Can you work these out from the model? Positions are in its coordinate system, mm. A direction names the side the tool comes from. Coordinates: 2 decimals unless noted, no trailing zeros. Loops run counter-clockwise (first coordinate to the right, second up) from the corner with the lowest first, then second, coordinate; pieces in that order, holes last. Notation, with made-up numbers: (-6.5, 38) -> (51.5, 38) arc R20 ccw to (51.5, 67) -> close; hole circle Ø7 at (-11.75, 21). An arc over 180 degrees is marked (long way). Use one line per item in the form item = value. Start each with the question number.
(1) On a 3-axis mill with a long thin cutter (end or side, diameter ignored), from which of +Z, -Z, +X, -X, +Y, -Y can I reach the whole of each face in a straight line? I mean faces 1 (the flat face through (3, -17.5, -124)), 2 (the cylindrical face through (-2.75, -92.74, 20.59)), 3 (the flat face through (3, 17.5, 124)). Say none if no direction works.
(2) Imagine slicing it at D-D (z = -121.5). List the corners of the cut face in (x, y) for me, plus the area to 3 significant figures.
(3) Thinking about a two-plate mould opening in Y: for faces 4 (the flat face through (3.41, 115.96, -46.74)), 5 (the flat face through (10, 59.85, 45.49)), 6 (the flat face through (0, 76, 0)), 7 (the cylindrical face through (3.409, 121.16, -60.934)), which applies, released by +Y, released by -Y, zero draft, split by the parting line, or undercut?
(4) I need wall thicknesses on line 1 (Y direction, x = 7.5, z = -62); line 2 (Y direction, x = 5, z = 75.5); line 3 (Y direction, x = -2.8, z = 0). Which ranges of each line are inside material? Lowest first, please. Write a range as [from, to].
(5) I'm going to push flat-ended pins straight in: pin 1 (4 mm diameter, centred on x = 6, z = -45.5, fed in from +Y); pin 2 (18.5 mm diameter, centred on y = 0, z = 133.66, fed in from -X); pin 3 (14.5 mm diameter, centred on y = 115.75, z = 66.83, fed in from -X); pin 4 (2 mm diameter, centred on y = -61.5, z = 56, fed in from -X). Where does each tip first touch, or does it pass through?
(6) Imagine slicing it at A-A (y = 0). List the corners of the cut face in (x, z) for me, plus the area to 3 significant figures.
(7) Imagine slicing it at C-C (x = 4.25). State how many separate pieces and enclosed holes the cut face has, plus the area to 3 significant figures.
(8) Imagine slicing it at B-B (z = 0). List the corners of the cut face in (x, y) for me, plus the area to 3 significant figures.
```python
from build123d import *

# Parameters (mm, degrees)
SKETCH2_R           = 115
SKETCH2_R_2         = 95
SKETCH2_R_3         = 75
SKETCH2_R_4         = 8
BOSS_EXTRUDE1_DEPTH = 10
BOSS_EXTRUDE2_START = -3
SKETCH2_5_R         = 115
SKETCH2_5_R_2       = 95
SKETCH2_5_R_3       = 8
BOSS_EXTRUDE2_DEPTH = 3
FILLET1_R           = 2.5


with BuildPart() as part:
    # Sketch2 → Boss-Extrude1 (new body)
    # profile 1 of 8: a face of its own
    with BuildSketch(Plane(origin=(0, 0, 0), x_dir=(0, 0, -1), z_dir=(1, 0, 0))):
        Circle(SKETCH2_R)
        Circle(SKETCH2_R_2, mode=Mode.SUBTRACT)
    # profile 2 of 8: a face of its own
    with BuildSketch(Plane(origin=(0, 0, 0), x_dir=(0, 0, -1), z_dir=(1, 0, 0))):
        Circle(SKETCH2_R_2)
        Circle(SKETCH2_R_3, mode=Mode.SUBTRACT)
    # profile 3 of 8: a face of its own
    with BuildSketch(Plane(origin=(0, 0, 0), x_dir=(0, 0, -1), z_dir=(1, 0, 0))):
        with BuildLine():
            ThreePointArc((-113.660679217, -17.5), (-115, 0), (-113.660679217, 17.5))
            Line((-113.660679217, 17.5), (-133.660679217, 17.5))
            ThreePointArc((-133.660679217, 17.5), (-151.160679217, 0), (-133.660679217, -17.5))
            Line((-133.660679217, -17.5), (-113.660679217, -17.5))
        make_face()
        with Locations((-133.660679217, 0)):
            Circle(SKETCH2_R_4, mode=Mode.SUBTRACT)
    # profile 4 of 8: a face of its own
    with BuildSketch(Plane(origin=(0, 0, 0), x_dir=(0, 0, -1), z_dir=(1, 0, 0))):
        with BuildLine():
            ThreePointArc((-71.985784175, 89.683035613), (-57.5, 99.592921435), (-41.674895042, 107.183035613))
            Line((-41.674895042, 107.183035613), (-51.674895042, 124.503543689))
            ThreePointArc((-51.674895042, 124.503543689), (-75.580339608, 130.908988255), (-81.985784175, 107.003543689))
            Line((-81.985784175, 107.003543689), (-71.985784175, 89.683035613))
        make_face()
        with Locations((-66.830339608, 115.753543689)):
            Circle(SKETCH2_R_4, mode=Mode.SUBTRACT)
    # profile 5 of 8: a face of its own
    with BuildSketch(Plane(origin=(0, 0, 0), x_dir=(0, 0, -1), z_dir=(1, 0, 0))):
        with BuildLine():
            ThreePointArc((41.674895042, 107.183035613), (57.5, 99.592921435), (71.985784175, 89.683035613))
            Line((71.985784175, 89.683035613), (81.985784175, 107.003543689))
            ThreePointArc((81.985784175, 107.003543689), (75.580339608, 130.908988255), (51.674895042, 124.503543689))
            Line((51.674895042, 124.503543689), (41.674895042, 107.183035613))
        make_face()
        with Locations((66.830339608, 115.753543689)):
            Circle(SKETCH2_R_4, mode=Mode.SUBTRACT)
    # profile 6 of 8: a face of its own
    with BuildSketch(Plane(origin=(0, 0, 0), x_dir=(0, 0, -1), z_dir=(1, 0, 0))):
        with BuildLine():
            Line((133.660679217, 17.5), (113.660679217, 17.5))
            ThreePointArc((113.660679217, 17.5), (114.66468094, 8.775588017), (115, 0))
            ThreePointArc((115, 0), (114.66468094, -8.775588017), (113.660679217, -17.5))
            Line((113.660679217, -17.5), (133.660679217, -17.5))
            ThreePointArc((133.660679217, -17.5), (151.160679217, 0), (133.660679217, 17.5))
        make_face()
        with Locations((133.660679217, 0)):
            Circle(SKETCH2_R_4, mode=Mode.SUBTRACT)
    # profile 7 of 8: a face of its own
    with BuildSketch(Plane(origin=(0, 0, 0), x_dir=(0, 0, -1), z_dir=(1, 0, 0))):
        with BuildLine():
            Line((81.985784175, -107.003543689), (71.985784175, -89.683035613))
            ThreePointArc((71.985784175, -89.683035613), (57.5, -99.592921435), (41.674895042, -107.183035613))
            Line((41.674895042, -107.183035613), (51.674895042, -124.503543689))
            ThreePointArc((51.674895042, -124.503543689), (75.580339608, -130.908988255), (81.985784175, -107.003543689))
        make_face()
        with Locations((66.830339608, -115.753543689)):
            Circle(SKETCH2_R_4, mode=Mode.SUBTRACT)
    # profile 8 of 8: a face of its own
    with BuildSketch(Plane(origin=(0, 0, 0), x_dir=(0, 0, -1), z_dir=(1, 0, 0))):
        with BuildLine():
            Line((-51.674895042, -124.503543689), (-41.674895042, -107.183035613))
            ThreePointArc((-41.674895042, -107.183035613), (-57.5, -99.592921435), (-71.985784175, -89.683035613))
            Line((-71.985784175, -89.683035613), (-81.985784175, -107.003543689))
            ThreePointArc((-81.985784175, -107.003543689), (-75.580339608, -130.908988255), (-51.674895042, -124.503543689))
        make_face()
        with Locations((-66.830339608, -115.753543689)):
            Circle(SKETCH2_R_4, mode=Mode.SUBTRACT)
    extrude(amount=BOSS_EXTRUDE1_DEPTH)

    # Sketch2_5 → Boss-Extrude2 (add)
    # profile 1 of 7: a face of its own
    with BuildSketch(Plane(origin=(0, 0, 0), x_dir=(0, 0, -1), z_dir=(1, 0, 0)).offset(BOSS_EXTRUDE2_START)):
        Circle(SKETCH2_5_R)
        Circle(SKETCH2_5_R_2, mode=Mode.SUBTRACT)
    # profile 2 of 7: a face of its own
    with BuildSketch(Plane(origin=(0, 0, 0), x_dir=(0, 0, -1), z_dir=(1, 0, 0)).offset(BOSS_EXTRUDE2_START)):
        with BuildLine():
            Line((133.660679217, 17.5), (113.660679217, 17.5))
            ThreePointArc((113.660679217, 17.5), (114.66468094, 8.775588017), (115, 0))
            ThreePointArc((115, 0), (114.66468094, -8.775588017), (113.660679217, -17.5))
            Line((113.660679217, -17.5), (133.660679217, -17.5))
            ThreePointArc((133.660679217, -17.5), (151.160679217, 0), (133.660679217, 17.5))
        make_face()
        with Locations((133.660679217, 0)):
            Circle(SKETCH2_5_R_3, mode=Mode.SUBTRACT)
    # profile 3 of 7: a face of its own
    with BuildSketch(Plane(origin=(0, 0, 0), x_dir=(0, 0, -1), z_dir=(1, 0, 0)).offset(BOSS_EXTRUDE2_START)):
        with BuildLine():
            ThreePointArc((41.674895042, 107.183035613), (57.5, 99.592921435), (71.985784175, 89.683035613))
            Line((71.985784175, 89.683035613), (81.985784175, 107.003543689))
            ThreePointArc((81.985784175, 107.003543689), (75.580339608, 130.908988255), (51.674895042, 124.503543689))
            Line((51.674895042, 124.503543689), (41.674895042, 107.183035613))
        make_face()
        with Locations((66.830339608, 115.753543689)):
            Circle(SKETCH2_5_R_3, mode=Mode.SUBTRACT)
    # profile 4 of 7: a face of its own
    with BuildSketch(Plane(origin=(0, 0, 0), x_dir=(0, 0, -1), z_dir=(1, 0, 0)).offset(BOSS_EXTRUDE2_START)):
        with BuildLine():
            ThreePointArc((-71.985784175, 89.683035613), (-57.5, 99.592921435), (-41.674895042, 107.183035613))
            Line((-41.674895042, 107.183035613), (-51.674895042, 124.503543689))
            ThreePointArc((-51.674895042, 124.503543689), (-75.580339608, 130.908988255), (-81.985784175, 107.003543689))
            Line((-81.985784175, 107.003543689), (-71.985784175, 89.683035613))
        make_face()
        with Locations((-66.830339608, 115.753543689)):
            Circle(SKETCH2_5_R_3, mode=Mode.SUBTRACT)
    # profile 5 of 7: a face of its own
    with BuildSketch(Plane(origin=(0, 0, 0), x_dir=(0, 0, -1), z_dir=(1, 0, 0)).offset(BOSS_EXTRUDE2_START)):
        with BuildLine():
            ThreePointArc((-113.660679217, -17.5), (-115, 0), (-113.660679217, 17.5))
            Line((-113.660679217, 17.5), (-133.660679217, 17.5))
            ThreePointArc((-133.660679217, 17.5), (-151.160679217, 0), (-133.660679217, -17.5))
            Line((-133.660679217, -17.5), (-113.660679217, -17.5))
        make_face()
        with Locations((-133.660679217, 0)):
            Circle(SKETCH2_5_R_3, mode=Mode.SUBTRACT)
    # profile 6 of 7: a face of its own
    with BuildSketch(Plane(origin=(0, 0, 0), x_dir=(0, 0, -1), z_dir=(1, 0, 0)).offset(BOSS_EXTRUDE2_START)):
        with BuildLine():
            Line((-51.674895042, -124.503543689), (-41.674895042, -107.183035613))
            ThreePointArc((-41.674895042, -107.183035613), (-57.5, -99.592921435), (-71.985784175, -89.683035613))
            Line((-71.985784175, -89.683035613), (-81.985784175, -107.003543689))
            ThreePointArc((-81.985784175, -107.003543689), (-75.580339608, -130.908988255), (-51.674895042, -124.503543689))
        make_face()
        with Locations((-66.830339608, -115.753543689)):
            Circle(SKETCH2_5_R_3, mode=Mode.SUBTRACT)
    # profile 7 of 7: a face of its own
    with BuildSketch(Plane(origin=(0, 0, 0), x_dir=(0, 0, -1), z_dir=(1, 0, 0)).offset(BOSS_EXTRUDE2_START)):
        with BuildLine():
            Line((81.985784175, -107.003543689), (71.985784175, -89.683035613))
            ThreePointArc((71.985784175, -89.683035613), (57.5, -99.592921435), (41.674895042, -107.183035613))
            Line((41.674895042, -107.183035613), (51.674895042, -124.503543689))
            ThreePointArc((51.674895042, -124.503543689), (75.580339608, -130.908988255), (81.985784175, -107.003543689))
        make_face()
        with Locations((66.830339608, -115.753543689)):
            Circle(SKETCH2_5_R_3, mode=Mode.SUBTRACT)
    extrude(amount=BOSS_EXTRUDE2_DEPTH)

    # Fillet1
    fillet1_edges = [part.edges().sort_by_distance(p)[0] for p in [
        (0, 0, 95),
    ]]
    fillet(fillet1_edges, radius=FILLET1_R)


solid = part.part
```
Worked out:
q1.face_1 = -Z, +X, -X, -Y
q1.face_2 = -X
q1.face_3 = +Z, +X, -X, +Y
q2.outline = (-3, -17.5) -> (10, -17.5) -> (10, 17.5) -> (-3, 17.5) -> close
q2.area = 455 mm2
q3.face_4 = released by +Y
q3.face_5 = zero draft
q3.face_6 = undercut
q3.face_7 = undercut
q4.line_1 = [-132.57, -122.13], [-109.38, -42.2], [42.2, 109.38], [122.13, 132.57]
q4.line_2 = [-130.96, -95.77], [-86.75, 86.75], [95.77, 130.96]
q4.line_3 = [-115, -95], [95, 115]
q5.pin_1 = 117.27
q5.pin_2 = -3
q5.pin_3 = through
q5.pin_4 = 0
q6.outline = (-3, -151.16) -> (10, -151.16) -> (10, -141.66) -> (-3, -141.66) -> close; (-3, -125.66) -> (10, -125.66) -> (10, -75) -> (0, -75) -> (0, -92.5) arc R2.5 cw to (-2.5, -95) -> (-3, -95) -> close; (-3, 95) -> (-2.5, 95) arc R2.5 cw to (0, 92.5) -> (0, 75) -> (10, 75) -> (10, 125.66) -> (-3, 125.66) -> close; (-3, 141.66) -> (10, 141.66) -> (10, 151.16) -> (-3, 151.16) -> close
q6.area = 1,450 mm2
q7.separate_pieces = 1
q7.enclosed_holes = 7
q7.area = 29,600 mm2
q8.outline = (-3, -115) -> (10, -115) -> (10, -75) -> (0, -75) -> (0, -92.5) arc R2.5 cw to (-2.5, -95) -> (-3, -95) -> close; (-3, 95) -> (-2.5, 95) arc R2.5 cw to (0, 92.5) -> (0, 75) -> (10, 75) -> (10, 115) -> (-3, 115) -> close
q8.area = 923 mm2
